The figure shows three views and two pictorial views of one solid part (mm, origin at its lowest corner). Answer the questions. Give positions to 0.01 mm unless a question says otherwise; leave off trailing zeros. Write each loop counter-clockwise with the first axis right and the second up, starting at its lowest first coordinate (ties: lowest second). Pieces come first, ordered by that corner, then holes. Notation, with made-up numbers: M 66.5,-35 L 86.5,-35 A26 ccw 86.5,2 Z; hole C -32,-38 d10. An arc over 180 degrees is marked long. Answer as CSV lines item,"result". Start each with the question number.
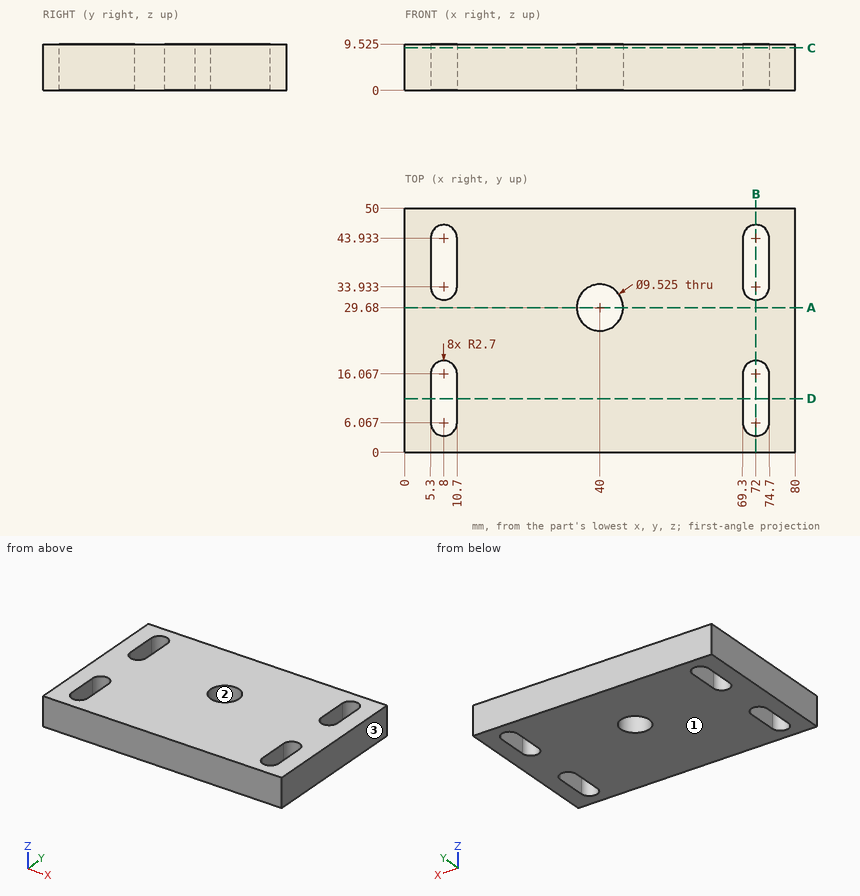
1. Find section C-C on z = 8.75. Determine the outline of the cut face in (x, y) (1 decimal).
2. Find section D-D on y = 11. Determine the outline of the cut face in (x, z) (3 decimals).
3. Find section B-B on x = 72. Determine the outline of the cut face in (y, z) (3 decimals).
4. Find section A-A on y = 29.68. Determine the outline of the cut face in (x, z) (1 decimal).
5. Find the intervals of material crossed by line 1 (X direction, y = 12.5, z = 6.75); line 2 (Y direction, x = 40, z = 3.75); line 3 (X direction, y = 17, z = 3), in increasing order. Write a range as [from, to].
6. Given pin 1 (3 mm diameter, centred on y = 9.5, z = 2.5, fed in from -X), flat-ended and moving along its own axis, determine where the tip first touches the part or whether it passes through.
7. Determine the mould class of the marked faces 1, 2 and 3 for opening direction X: +X half, -X half, draft (parallel to the pull), parting line (faces both ways), or undercut.
Computed:
1,outline,"M 0,0 L 80,0 L 80,50 L 0,50 Z; hole M 5.3,6.1 A2.7 ccw 10.7,6.1 L 10.7,16.1 A2.7 ccw 5.3,16.1 Z; hole M 5.3,33.9 A2.7 ccw 10.7,33.9 L 10.7,43.9 A2.7 ccw 5.3,43.9 Z; hole C 40,29.7 d9.5; hole M 69.3,6.1 A2.7 ccw 74.7,6.1 L 74.7,16.1 A2.7 ccw 69.3,16.1 Z; hole M 69.3,33.9 A2.7 ccw 74.7,33.9 L 74.7,43.9 A2.7 ccw 69.3,43.9 Z"
2,outline,"M 0,0 L 5.3,0 L 5.3,9.525 L 0,9.525 Z; M 10.7,0 L 69.3,0 L 69.3,9.525 L 10.7,9.525 Z; M 74.7,0 L 80,0 L 80,9.525 L 74.7,9.525 Z"
3,outline,"M 0,0 L 3.367,0 L 3.367,9.525 L 0,9.525 Z; M 18.767,0 L 31.233,0 L 31.233,9.525 L 18.767,9.525 Z; M 46.633,0 L 50,0 L 50,9.525 L 46.633,9.525 Z"
4,outline,"M 0,0 L 35.2,0 L 35.2,9.5 L 0,9.5 Z; M 44.8,0 L 80,0 L 80,9.5 L 44.8,9.5 Z"
5,line 1,"x = [0, 5.3], [10.7, 69.3], [74.7, 80]"
5,line 2,"y = [0, 24.92], [34.44, 50]"
5,line 3,"x = [0, 5.47], [10.53, 69.47], [74.53, 80]"
6,pin 1,"stops at x = 0"
7,face 1,"draft"
7,face 2,"undercut"
7,face 3,"+X half"
